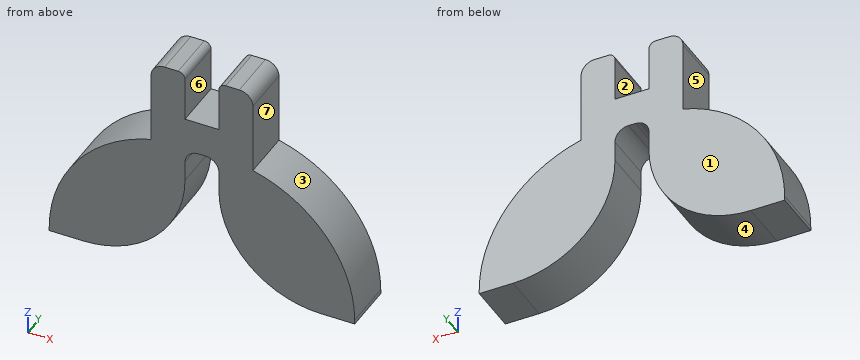
from build123d import *

# Parameters (mm, degrees)
F0_W        = 6.35
F0_H        = 12.7
F1_DEPTH    = 19.05
F2_R        = 2.54
F3_R        = 38.1
F4_T1_DEPTH = 264.9844424842
F5_R        = 5.08
F6_R        = 5.08


# Not quite as in the source:
# - a fillet or chamfer that OpenCascade refuses, or shapes differently, is made with other operations: its cross-section is extruded or revolved along the edge and cut away or added


with BuildPart() as f1:
    # F0 (on Front) → F1 (new body)
    with BuildSketch(Plane.XZ):
        Polygon((-6.35, -50.8), (-6.35, 0), (-19.05, 0), (-57.15, 0), (-57.15, -50.8), align=None)
        Polygon((-19.05, 0), (-6.35, 0), (-6.35, 12.7), (-6.35, 31.75), (-19.05, 31.75), align=None)
        with Locations((-3.175, 6.35)):
            Rectangle(F0_W, F0_H)
        with Locations((3.175, 6.35)):
            Rectangle(F0_W, F0_H)
        Polygon((6.35, 12.7), (6.35, 0), (19.05, 0), (19.05, 31.75), (6.35, 31.75), align=None)
        Polygon((19.05, 0), (6.35, 0), (6.35, -50.8), (57.15, -50.8), (57.15, 0), align=None)
    extrude(amount=F1_DEPTH)

    # F2
    f2_edges = [f1.edges().sort_by_distance(p)[0] for p in [
        (6.35, -9.525, 31.75),
        (-6.35, -9.525, 31.75),
    ]]
    fillet(f2_edges, radius=F2_R)

    # F3
    f3_edges = [f1.edges().sort_by_distance(p)[0] for p in [
        (6.35, -9.525, -50.8),
        (-6.35, -9.525, -50.8),
    ]]
    fillet(f3_edges, radius=F3_R)

    # F4: fillet of radius 50.8 on 2 edges, made by hand

    # F4_s2 → F4_t1 (cut)
    with BuildSketch(Plane.XZ.offset(-122.9672212421)):
        with BuildLine():
            ThreePointArc((-57.15, -49.1868884968), (-46.5109262841, -18.0783687635), (-19.05, 0))
            Line((-19.05, 0), (-57.15, 0))
            Line((-57.15, 0), (-57.15, -49.1868884968))
        make_face()
        with BuildLine():
            ThreePointArc((57.15, -49.1868884968), (46.5109262841, -18.0783687635), (19.05, 0))
            Line((19.05, 0), (57.15, 0))
            Line((57.15, 0), (57.15, -49.1868884968))
        make_face()
    extrude(amount=F4_T1_DEPTH, mode=Mode.SUBTRACT)

    # F5
    f5_edges = [f1.edges().sort_by_distance(p)[0] for p in [
        (-19.05, -9.525, 31.75),
        (19.05, -9.525, 31.75),
    ]]
    fillet(f5_edges, radius=F5_R)

    # F6
    f6_edges = [f1.edges().sort_by_distance(p)[0] for p in [
        (6.35, -9.525, 0),
        (-6.35, -9.525, 0),
    ]]
    fillet(f6_edges, radius=F6_R)


solid = f1.part
For this review, take the finished solid that the model builds, in its own axes (mm). Face numbers are marked on the shaded views. A direction names the side the tool comes from. Give positions to 0.01 mm unless a question says otherwise; leave off trailing zeros. Loops run counter-clockwise (first coordinate to the right, second up) from the corner with the lowest first, then second, coordinate; pieces in that order, holes last.
Item 1: Draft analysis for pull direction X (two halves, no side actions). For the marked faces 1, 2, 3 and 4, state which applies: +X half, -X half, draft (parallel to the pull), parting line (faces both ways), or undercut.
Item 2: Take a section at C-C, the plane z = -32.5. State the section outline as (x, y) points, and give its area (3 significant figures).
Item 3: Take a section at A-A, the plane z = 15.5. State the section outline as (x, y) points, and give its area (3 significant figures).
Item 4: For line 1 along X through (y, z) = (-14, 21.5); line 2 along X through (y, z) = (-14.5, 4.5); line 3 along X through (y, z) = (-13.75, -41.5), list the stretches that pass through material, from the lowest coordinate up.
Item 5: Insertion check: pin 1 (4 mm diameter, centred on y = -13, z = -20.5, fed in from +X); pin 2 (8 mm diameter, centred on x = 8, y = -13.5, fed in from -Z); pin 3 (10 mm diameter, centred on x = 3, y = -9, fed in from +Z). Each pin has a flat end and moves straight along its axis. Give the tip position at first contact, or say it passes through.
Item 6: Take a section at B-B, the plane y = -15.5. State the section outline as (x, z) points, and give its area (3 significant figures).
Item 7: Take a section at D-D, the plane x = -27.5. State the section outline as (y, z) points, and give its area (3 significant figures).
Item 8: Tool access review of the marked faces 5, 6 and 7: name each direction out of +Z, -Z, +X, -X, +Y, -Y from which nothing blocks a thin tool from reaching the whole face with its end or side.
Calculated:
1. face 1: draft
1. face 2: undercut
1. face 3: +X half
1. face 4: undercut
2. outline: (-54.33, -19.05) - (-11.9, -19.05) - (-11.9, 0) - (-54.33, 0) - close; (11.9, -19.05) - (54.33, -19.05) - (54.33, 0) - (11.9, 0) - close
2. area: 1,620 mm2
3. outline: (-19.05, -19.05) - (-6.35, -19.05) - (-6.35, 0) - (-19.05, 0) - close; (6.35, -19.05) - (19.05, -19.05) - (19.05, 0) - (6.35, 0) - close
3. area: 484 mm2
4. line 1: x = -19.05 to -6.35, 6.35 to 19.05
4. line 2: x = -19.05 to 19.05
4. line 3: x = -56.57 to -19.51, 19.51 to 56.57
5. pin 1: stops at x = 49.58
5. pin 2: stops at z = -32.67
5. pin 3: stops at z = 31.59
6. outline: (-57.15, -50.8) - (-44.45, -50.8) arc R38.1 ccw to (-6.35, -12.7) - (-6.35, -5.08) arc R5.08 cw to (-1.27, 0) - (1.27, 0) arc R5.08 cw to (6.35, -5.08) - (6.35, -12.7) arc R38.1 ccw to (44.45, -50.8) - (57.15, -50.8) - (57.15, -49.19) arc R50.8 ccw to (19.05, 0) - (19.05, 26.67) arc R5.08 ccw to (13.97, 31.75) - (8.89, 31.75) arc R2.54 ccw to (6.35, 29.21) - (6.35, 12.7) - (-6.35, 12.7) - (-6.35, 29.21) arc R2.54 ccw to (-8.89, 31.75) - (-13.97, 31.75) arc R5.08 ccw to (-19.05, 26.67) - (-19.05, 0) arc R50.8 ccw to (-57.15, -49.19) - close
6. area: 4,530 mm2
7. outline: (-19.05, -46.82) - (0, -46.82) - (0, -3) - (-19.05, -3) - close
7. area: 835 mm2
8. face 5: +Z, -X, +Y, -Y
8. face 6: +Z, +Y, -Y
8. face 7: +Z, +X, +Y, -Y
